```python
from build123d import *

# Parameters (mm, degrees)
SKETCH1_W               = 50
SKETCH1_H               = 12.5
SKETCH1_W_2             = 5
BOSS_EXTRUDE1_DEPTH     = 12.5
FILLET1_R               = 6.25
CUT_EXTRUDE1_DEPTH      = 77.5
CUT_EXTRUDE1_DEPTH_BACK = 24.5
SKETCH2_R               = 2.5
SKETCH4_R               = 1.25
CUT_EXTRUDE2_DEPTH      = 12.5
BOSS_EXTRUDE4_DEPTH     = 6
BOSS_EXTRUDE5_DEPTH     = 5
BOSS_EXTRUDE6_DEPTH     = 5
BOSS_EXTRUDE8_DEPTH     = 6.75
BOSS_EXTRUDE10_DEPTH    = 55
SKETCH12_W              = 2.5
SKETCH12_H              = 10
BOSS_EXTRUDE11_DEPTH    = 11.25
SKETCH14_W              = 2.5
SKETCH14_H              = 10
BOSS_EXTRUDE12_DEPTH    = 11.25
FILLET2_R               = 5.625
SKETCH16_R              = 1.75
CUT_EXTRUDE3_DEPTH      = 18.25


with BuildPart() as part:
    # Sketch1 → Boss-Extrude1 (new body)
    with BuildSketch(Plane.XY):
        with Locations((25, -6.25)):
            Rectangle(SKETCH1_W, SKETCH1_H)
        with Locations((2.5, -18.75)):
            Rectangle(SKETCH1_W_2, SKETCH1_H)
        with Locations((47.5, -18.75)):
            Rectangle(SKETCH1_W_2, SKETCH1_H)
    extrude(amount=BOSS_EXTRUDE1_DEPTH)

    # Fillet1
    fillet1_edges = [part.edges().sort_by_distance(p)[0] for p in [
        (2.5, -25, 12.5),
        (2.5, -25, 0),
        (47.5, -25, 12.5),
        (47.5, -25, 0),
    ]]
    fillet(fillet1_edges, radius=FILLET1_R - 0.0001)  # a hair under: the kernel refuses the full size

    # Sketch2 → Cut-Extrude1 (cut, two sides: drawn at the far end of the back side and taken through both)
    with BuildSketch(Plane(origin=(5, 0, 0), x_dir=(0, 0, -1), z_dir=(1, 0, 0)).offset(-CUT_EXTRUDE1_DEPTH_BACK)):
        with Locations((-6.25, -18.75)):
            Circle(SKETCH2_R)
    extrude(amount=CUT_EXTRUDE1_DEPTH + CUT_EXTRUDE1_DEPTH_BACK, mode=Mode.SUBTRACT)

    # Sketch4 → Cut-Extrude2 (cut)
    with BuildSketch(Plane(origin=(0, -12.5, 0), x_dir=(-1, 0, 0), z_dir=(0, -1, 0))):
        with Locations(Location((-8, -9.835613506, 0), (0, 0, 90))):
            Circle(SKETCH4_R)
        with Locations(Location((-15, -9.835613506, 0), (0, 0, 90))):
            Circle(SKETCH4_R)
        with Locations(Location((-25, -9.835613506, 0), (0, 0, 90))):
            Circle(SKETCH4_R)
        with Locations(Location((-35, -9.835613506, 0), (0, 0, 90))):
            Circle(SKETCH4_R)
        with Locations(Location((-42, -9.835613506, 0), (0, 0, 90))):
            Circle(SKETCH4_R)
    extrude(amount=-CUT_EXTRUDE2_DEPTH, mode=Mode.SUBTRACT)

    # Sketch5 → Boss-Extrude4 (add)
    with BuildSketch(Plane(origin=(0, 0, 0), x_dir=(1, 0, 0), z_dir=(0, 1, 0))):
        Polygon((50, 0), (0, 0), (0, -6.75), (5.75, -6.75), (44.25, -6.75), (50, -6.75), align=None)
    extrude(amount=BOSS_EXTRUDE4_DEPTH)

    # Sketch6 → Boss-Extrude5 (add)
    with BuildSketch(Plane.ZY):
        Polygon((6.75, 6), (12.5, 0), (6.75, 0), align=None)
    extrude(amount=-BOSS_EXTRUDE5_DEPTH)

    # Sketch7 → Boss-Extrude6 (add)
    with BuildSketch(Plane(origin=(50, 0, 0), x_dir=(0, 0, -1), z_dir=(1, 0, 0))):
        Polygon((-6.75, 6), (-12.5, 0), (-6.75, 0), align=None)
    extrude(amount=-BOSS_EXTRUDE6_DEPTH)

    # Sketch8 → Boss-Extrude8 (add)
    with BuildSketch(Plane(origin=(0, 0, 0), x_dir=(-1, 0, 0), z_dir=(0, 0, -1))):
        Polygon((-50, 6), (-55, 14.660254038), (-55, 64.660254038), (0, 64.660254038), (0, 6), align=None)
    extrude(amount=-BOSS_EXTRUDE8_DEPTH)

    # Sketch10 → Boss-Extrude10 (add)
    with BuildSketch(Plane.ZY):
        Polygon((6.75, 64.660254038), (11.25, 64.660254038), (6.75, 60.225702909), align=None)
    extrude(amount=-BOSS_EXTRUDE10_DEPTH)

    # Sketch12 → Boss-Extrude11 (add)
    with BuildSketch(Plane(origin=(0, 0, 0), x_dir=(-1, 0, 0), z_dir=(0, 0, -1))):
        with Locations((-1.25, 69.660254038)):
            Rectangle(SKETCH12_W, SKETCH12_H)
    extrude(amount=-BOSS_EXTRUDE11_DEPTH)

    # Sketch14 → Boss-Extrude12 (add)
    with BuildSketch(Plane(origin=(0, 0, 0), x_dir=(-1, 0, 0), z_dir=(0, 0, -1))):
        with Locations((-7.75, 69.660254038)):
            Rectangle(SKETCH14_W, SKETCH14_H)
    extrude(amount=-BOSS_EXTRUDE12_DEPTH)

    # Fillet2
    fillet2_edges = [part.edges().sort_by_distance(p)[0] for p in [
        (7.75, 74.660254038, 0),
        (7.75, 74.660254038, 11.25),
        (1.25, 74.660254038, 11.25),
        (1.25, 74.660254038, 0),
    ]]
    fillet(fillet2_edges, radius=FILLET2_R - 0.0001)  # a hair under: the kernel refuses the full size

    # Sketch16 → Cut-Extrude3 (cut)
    with BuildSketch(Plane(origin=(9, 0, 0), x_dir=(0, 0, -1), z_dir=(1, 0, 0))):
        with Locations(Location((-5.625, 69.660254038, 0), (0, 0, 90))):
            Circle(SKETCH16_R)
    extrude(amount=-CUT_EXTRUDE3_DEPTH, mode=Mode.SUBTRACT)


solid = part.part
```
The model under review builds one solid part; all positions refer to its coordinate system, in mm. A direction names the side the tool comes from. Give positions to 0.01 mm unless a question says otherwise; leave off trailing zeros. Write each loop counter-clockwise with the first axis right and the second up, starting at its lowest first coordinate (ties: lowest second). Pieces come first, ordered by that corner, then holes.
(1) Tool access review of faces 1 (the flat face through (6.5, 68, 4)), 2 (the flat face through (25, 0, 8)), 3 (the flat face through (32, 64.66, 6)), 4 (the cylindrical face through (7.52, -6.34, 8.68)), 5 (the flat face through (45, -16, 6)): name each direction out of +Z, -Z, +X, -X, +Y, -Y from which nothing blocks a thin tool from reaching the whole face with its end or side.
(2) To check wall thickness, follow L1, parallel to Y at x = 46.4, z = 6.25; L2, parallel to Z at x = 47.05, y = -18.75; L3, parallel to Y at x = 2.2, z = 6.25. State the ranges of each line that lie inside material, in increasing order.
(3) Consider section D-D, the plane y = 21. Give the boundary of the cut face in (x, z).
(4) The part is to be moulded in two halves that separate along Y. For faces 6 (the flat face through (55, 40, 3)), 7 (the cylindrical face through (47.54, -23.22, 10.62)), 8 (the flat face through (2.465, 3.042, 9.585)), say which applies: released by +Y, released by -Y, zero draft, split by the parting line, or undercut.
(5) For P1, Ø6, axis at y = -18.75, z = 6.25, coming from the -X side; P2, Ø4, axis at x = 8, z = 9.84, coming from the +Y side; P3, Ø1.5, axis at y = 13, z = 1.5, coming from the +X side; P4, Ø3, axis at x = 18.5, z = 10.5, coming from the +Y side, all flat-tipped, find the tip position at first contact; note any pin that passes through.
(6) Consider section B-B, the plane x = 8. Give the number of separate pieces and of enclosed holes in the cut face, and give its area (3 significant figures).
(7) Consider section A-A, the plane x = 15. Give the boundary of the cut face in (y, z), and give its area (3 significant figures).
(8) Consider section C-C, the plane y = -3. Give the boundary of the cut face in (x, z), and give its area (3 significant figures).
Returned:
1. face 1: +Z, -Z, +Y
1. face 2: +Z
1. face 3: +Z, -Z, +X, +Y
1. face 4: -Y
1. face 5: +Z, -Z, -Y
2. L1: y = -25 to -21.25, -16.25 to 64.66
2. L2: z = 0 to 3.75, 8.75 to 12.5
2. L3: y = -25 to -21.25, -16.25 to 68.03, 71.29 to 74.63
3. outline: (0, 0) - (55, 0) - (55, 6.75) - (0, 6.75) - close
4. face 6: zero draft
4. face 7: released by -Y
4. face 8: undercut
5. P1: stops at x = 0
5. P2: stops at y = 74.21
5. P3: stops at x = 54.47
5. P4: stops at y = 64.66
6. separate pieces: 2
6. enclosed holes: 1
6. area: 661 mm2
7. outline: (-12.5, 0) - (64.66, 0) - (64.66, 11.25) - (60.23, 6.75) - (0, 6.75) - (0, 8.59) - (-12.5, 8.59) - close; (-12.5, 11.09) - (0, 11.09) - (0, 12.5) - (-12.5, 12.5) - close
7. area: 571 mm2
8. outline: (0, 0) - (50, 0) - (50, 12.5) - (0, 12.5) - close; hole circle Ø2.5 at (8, 9.84); hole circle Ø2.5 at (15, 9.84); hole circle Ø2.5 at (25, 9.84); hole circle Ø2.5 at (35, 9.84); hole circle Ø2.5 at (42, 9.84)
8. area: 600 mm2
